Autodesk Inventor part; units mm, degrees
ref_plane "YZ Plane" through (0, 0, 0) normal (1, 0, 0) x (0, 1, 0)
ref_plane "XZ Plane" through (0, 0, 0) normal (0, 1, 0) x (-1, 0, 0)
ref_plane "XY Plane" through (0, 0, 0) normal (0, 0, 1) x (1, 0, 0)
sketch "Sketch1" plane through (0, 0, 0) normal (0, 1, 0) x (-1, 0, 0)
  line L0 (16.5354, 24.0815) -> (16.5354, -24.0815)
  arc A0 (16.5354, 24.0815) -> (13.8037, 25.213) centre (14.9352, 24.0815) ccw
  line L1 (0, 11.4094) -> (13.8037, 25.213)
  line L2 (0, -11.4094) -> (0, 11.4094)
  line L3 (13.8037, -25.213) -> (0, -11.4094)
  arc A1 (13.8037, -25.213) -> (16.5354, -24.0815) centre (14.9352, -24.0815) ccw
  line L4 (-16.5354, 24.0815) -> (-16.5354, -24.0815)
  arc A2 (-13.8037, 25.213) -> (-16.5354, 24.0815) centre (-14.9352, 24.0815) ccw
  line L5 (0, 11.4094) -> (-13.8037, 25.213)
  line L6 (-13.8037, -25.213) -> (0, -11.4094)
  arc A3 (-16.5354, -24.0815) -> (-13.8037, -25.213) centre (-14.9352, -24.0815) ccw
  line L7 (16.3854, 24.063) -> (16.3854, -24.063)
  arc A4 (16.3854, 24.063) -> (13.8967, 25.0939) centre (14.9275, 24.063) ccw
  line L8 (0, 11.1972) -> (13.8967, 25.0939)
  line L9 (0, -11.1972) -> (0, 11.1972)
  line L10 (13.8967, -25.0939) -> (0, -11.1972)
  arc A5 (13.8967, -25.0939) -> (16.3854, -24.063) centre (14.9275, -24.063) ccw
  line L11 (-16.3854, 24.063) -> (-16.3854, -24.063)
  arc A6 (-13.8967, 25.0939) -> (-16.3854, 24.063) centre (-14.9275, 24.063) ccw
  line L12 (0, 11.1972) -> (-13.8967, 25.0939)
  line L13 (-13.8967, -25.0939) -> (0, -11.1972)
  arc A7 (-16.3854, -24.063) -> (-13.8967, -25.0939) centre (-14.9275, -24.063) ccw
  point P0 (0, 0)
  point P1 (0, 0)
  point P2 (0, 0)
  point P3 (15.5476, -25.5599)
  point P4 (15.4854, -25.4099)
  dimension "d3" = 1.6002
  dimension "d4" = 33.0708
  dimension "d5" = 16.1353
  dimension "d6" = 0.15
  dimension "d7" = 0.15
  dimension "d8" = 0.15
extrude "Extrusion1" add sketch "Sketch1" along normal blind 19.05 contours L8 A4 L7 A5 L10 L2 | L2 L13 A7 L11 A6 L12
properties part number "IPT_Dovetail_Connecter" material "Acetal Resin, Black"
Source: CAD feature listing. Evaluate the final solid. Frame: model axes, mm. A direction names the side the tool comes from. Round coordinates to 2 decimals unless told otherwise and drop trailing zeros. Loops run counter-clockwise (first coordinate to the right, second up) from the corner with the lowest first, then second, coordinate; pieces in that order, holes last.
Q1. Section A-A, the plane z = 22.5. Return loops of the section in (x, y), plus the area to 3 significant figures.
Q2. Section D-D, the plane x = 7. Return loops of the section in (y, z).
Q3. Section B-B, the plane y = 4. Return loops of the section in (x, z).
Q4. Mould query, pull axis X, two halves, no side actions, for faces 4 (the face through (16.385, 9, 0)), 5 (the face through (-15.46, 9.39, 25.42)), 6 (the face through (0, 0, 0)), 7 (the face through (15.51, 9.39, 25.4)). Classes: pulls with the +X half, pulls with the -X half, needs draft (parallel to the pull), parting line crosses it, or undercut.
Q5. Section C-C, the plane z = 15. Return loops of the section in (x, y).
Q6. Ray query, line 1 (X direction, y = 15.25, z = -15.5); line 2 (X direction, y = 12.5, z = -17); line 3 (Z direction, x = -1.5, y = 12.5). Return the intervals inside material, ascending.
Q7. First-contact query: P1, Ø10, axis at x = 3.5, y = 16, coming from the +Z side; P2, Ø4, axis at x = 10.5, y = 15.5, coming from the +Z side; P3, Ø6, axis at x = 11.5, y = 12.5, coming from the -Z side. Flat tips, straight axial feed; report the tip coordinate or a pass-through.
Q8. Access query for faces 1 (the face through (-7, 9.4, -18.2)), 2 (the face through (0, 19.05, 0)), 3 (the face through (6.85, 9.39, 18.05)). Directions: +Z, -Z, +X, -X, +Y, -Y. A direction counts if a zero-diameter tool reaches every point of the face in a straight line with its end or side. Return the directions, or none.
Solutions:
1. outline: (-16.39, 0) - (-11.3, 0) - (-11.3, 19.05) - (-16.39, 19.05) - close; (11.3, 0) - (16.39, 0) - (16.39, 19.05) - (11.3, 19.05) - close
1. area: 194 mm2
2. outline: (0, -18.2) - (19.05, -18.2) - (19.05, 18.2) - (0, 18.2) - close
3. outline: (-16.39, -24.06) arc R1.46 ccw to (-13.9, -25.09) - (0, -11.2) - (13.9, -25.09) arc R1.46 ccw to (16.39, -24.06) - (16.39, 24.06) arc R1.46 ccw to (13.9, 25.09) - (0, 11.2) - (-13.9, 25.09) arc R1.46 ccw to (-16.39, 24.06) - close
4. face 4: pulls with the +X half
4. face 5: undercut
4. face 6: needs draft
4. face 7: undercut
5. outline: (-16.39, 0) - (-3.8, 0) - (-3.8, 19.05) - (-16.39, 19.05) - close; (3.8, 0) - (16.39, 0) - (16.39, 19.05) - (3.8, 19.05) - close
6. line 1: x = -16.39 to -4.3, 4.3 to 16.39
6. line 2: x = -16.39 to -5.8, 5.8 to 16.39
6. line 3: z = -12.7 to 12.7
7. P1: stops at z = 19.7
7. P2: stops at z = 23.7
7. P3: stops at z = -25.46
8. face 1: -Z, +Y, -Y
8. face 2: +Z, -Z, +X, -X, +Y
8. face 3: +Z, +Y, -Y
